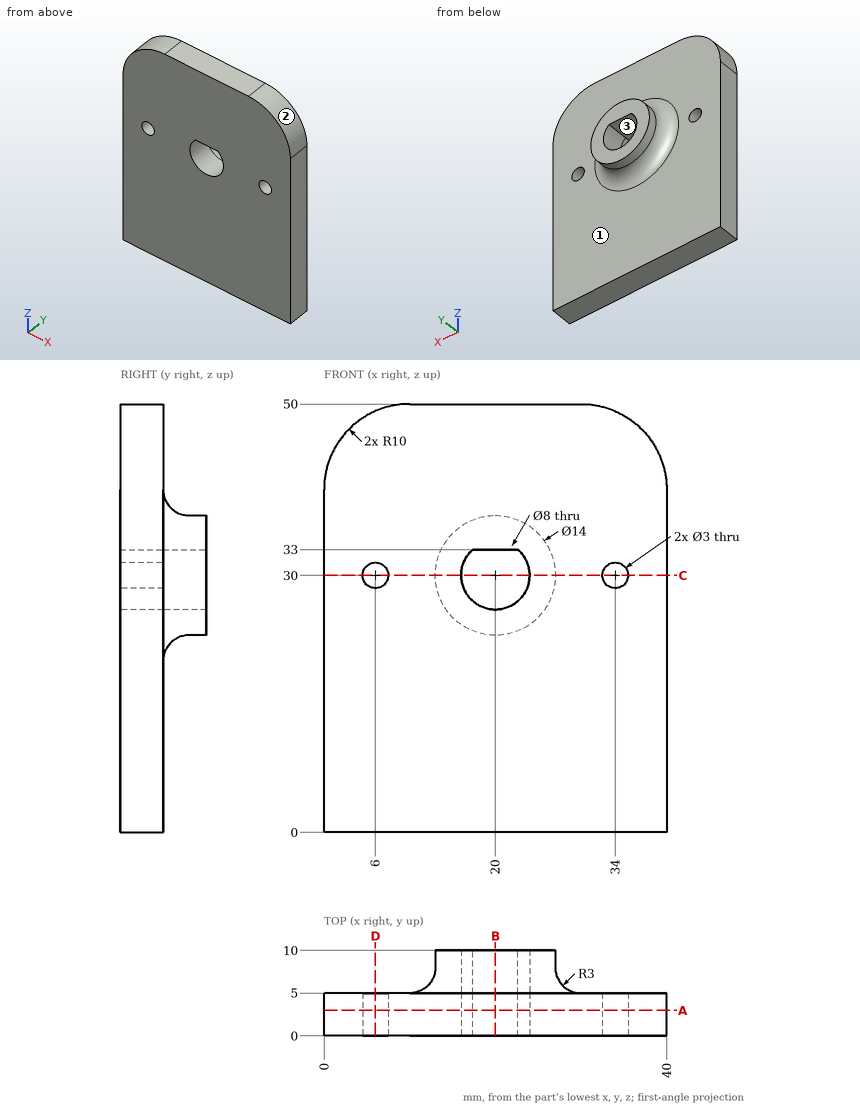
Verification items for this drawing (mm, ordinates from the low corner). Coordinates: 2 decimals unless noted, no trailing zeros. Order: outer loops, then holes, each group sorted by start corner. A loop starts at its lowest first (then second) coordinate and runs counter-clockwise, first axis right, second up.
Q1. Sectioned sample at D-D on x = 6. Record the cut outline in (y, z).
Reply:
outline: (0, 0) - (5, 0) - (5, 28.5) - (0, 28.5) - close; (0, 31.5) - (5, 31.5) - (5, 49.17) - (0, 49.17) - close
Q2. Sectioned sample at C-C on z = 30. Record the cut outline in (x, y).
Reply:
outline: (0, 0) - (4.5, 0) - (4.5, 5) - (0, 5) - close; (7.5, 0) - (16, 0) - (16, 10) - (13, 10) - (13, 8) arc R3 cw to (10, 5) - (7.5, 5) - close; (24, 0) - (32.5, 0) - (32.5, 5) - (30, 5) arc R3 cw to (27, 8) - (27, 10) - (24, 10) - close; (35.5, 0) - (40, 0) - (40, 5) - (35.5, 5) - close
Q3. Sectioned sample at A-A on y = 3. Record the cut outline in (x, z).
Reply:
outline: (0, 0) - (40, 0) - (40, 40) arc R10 ccw to (30, 50) - (10, 50) arc R10 ccw to (0, 40) - close; hole circle Ø3 at (6, 30); hole (17.35, 33) arc R4 ccw (long way) to (22.65, 33) - close; hole circle Ø3 at (34, 30)
Q4. Thickness scan on probe 1 along X at (y, z) = (2.05, 30); probe 2 along X at (y, z) = (8.7, 30); probe 3 along Z at (x, y) = (20, 1.75). Record the ranges inside material, lowest first.
Reply:
probe 1: x = 0 to 4.5, 7.5 to 16, 24 to 32.5, 35.5 to 40
probe 2: x = 13 to 16, 24 to 27
probe 3: z = 0 to 26, 33 to 50
Q5. Draft check along Z on the marked faces 1, 2 and 3. Enter one of: released by +Z, released by -Z, zero draft, split by the parting line, or undercut.
Reply:
face 1: zero draft
face 2: released by +Z
face 3: undercut
Q6. Depth check by flat-ended pin: pin 1 Ø10.5 at (x, z) = (20, 30) entering from -Y; pin 2 Ø1.6 at (x, y) = (21, 7) entering from -Z. Enter the tip coordinate at first touch or a pass-through.
Reply:
pin 1: stops at y = 0
pin 2: stops at z = 22.46
Q7. Sectioned sample at B-B on x = 20. Record the cut outline in (y, z).
Reply:
outline: (0, 0) - (5, 0) - (5, 20) arc R3 cw to (8, 23) - (10, 23) - (10, 26) - (0, 26) - close; (0, 33) - (10, 33) - (10, 37) - (8, 37) arc R3 cw to (5, 40) - (5, 50) - (0, 50) - close
